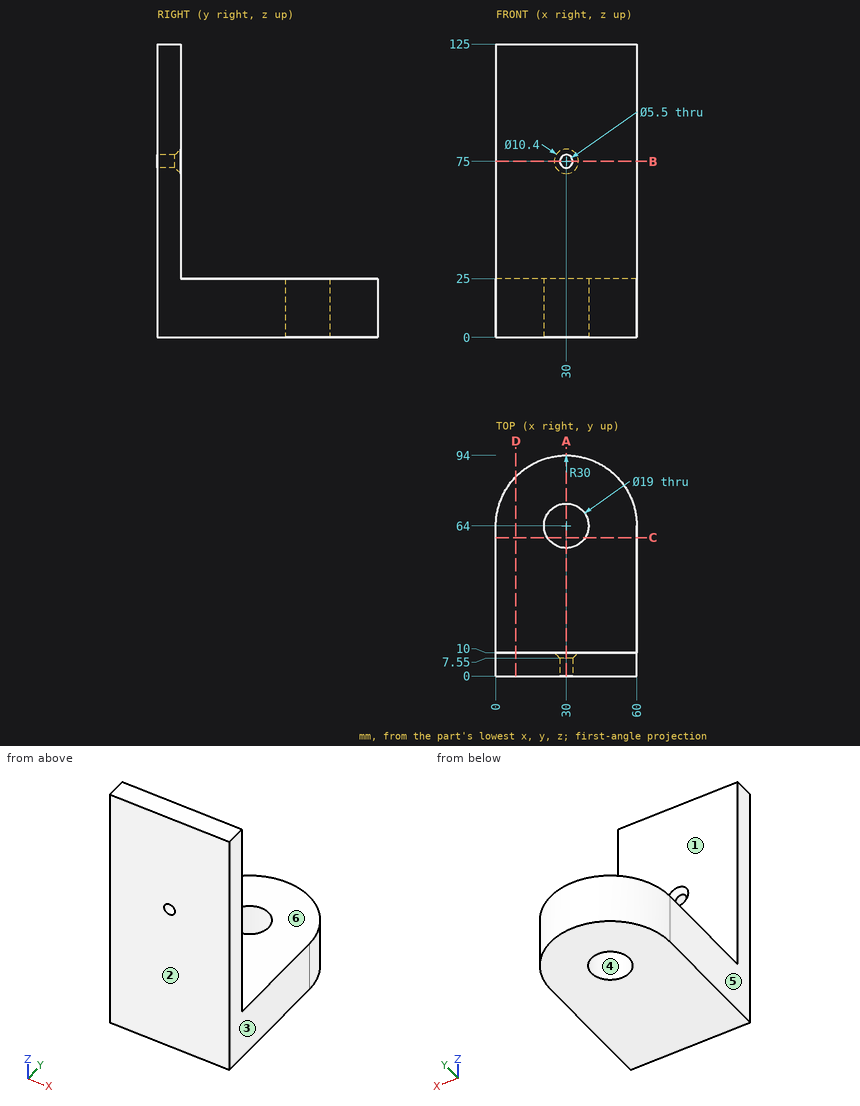
Input: dimensioned drawing with shaded views. Units: mm. Origin: part minimum x, y, z. A direction names the side the tool comes from. Round coordinates to 2 decimals unless told otherwise and drop trailing zeros. Order: outer loops, then holes, each group sorted by start corner. A loop starts at its lowest first (then second) coordinate and runs counter-clockwise, first axis right, second up.
1. Cut plane B-B, the plane z = 75. Output: boundary loops of the cut face in (x, y).
The answers:
outline: (0, 0) - (27.25, 0) - (27.25, 7.55) - (24.8, 10) - (0, 10) - close; (32.75, 0) - (60, 0) - (60, 10) - (35.2, 10) - (32.75, 7.55) - close
2. Cut plane C-C, the plane y = 59. Output: boundary loops of the cut face in (x, z), then the cut area to 3 significant figures.
The answers:
outline: (0, 0) - (21.92, 0) - (21.92, 25) - (0, 25) - close; (38.08, 0) - (60, 0) - (60, 25) - (38.08, 25) - close
area: 1,100 mm2
3. Pin query (flat end, axial travel): P1, Ø12, axis at x = 37.5, y = 82, coming from the +Z side; P2, Ø3, axis at x = 42.5, z = 53, coming from the +Y side; P3, Ø1.5, axis at x = 22, y = 51.5, coming from the -Z side; P4, Ø5, axis at y = 72.5, z = 18.5, coming from the +X side. Return the tip coordinate at first contact, or that it passes through.
The answers:
P1: stops at z = 25
P2: stops at y = 10
P3: stops at z = 0
P4: stops at x = 59.39
4. Mould query, pull axis Y, two halves, no side actions, for the marked faces 1, 2, 3 and 4. Classes: released by +Y, released by -Y, zero draft, split by the parting line, or undercut.
The answers:
face 1: released by +Y
face 2: released by -Y
face 3: zero draft
face 4: undercut
5. Cut plane D-D, the plane x = 8.5. Output: boundary loops of the cut face in (y, z), then the cut area to 3 significant figures.
The answers:
outline: (0, 0) - (84.92, 0) - (84.92, 25) - (10, 25) - (10, 125) - (0, 125) - close
area: 3,120 mm2
6. Set-up query: the marked faces 5 and 6. Return all of +Z, -Z, +X, -X, +Y, -Y with unobstructed straight access to the full face (end or side cutting, diameter ignored); none if empty.
The answers:
face 5: +Z, -Z, -X, +Y, -Y
face 6: +Z, +X, -X, +Y
7. Material intervals for line 1 (X direction, y = 2, z = 75); line 2 (Y direction, x = 30, z = 5); line 3 (Z direction, x = 30, y = 2.25), sorted ascending.
The answers:
line 1: x = 0 to 27.25, 32.75 to 60
line 2: y = 0 to 54.5, 73.5 to 94
line 3: z = 0 to 72.25, 77.75 to 125
8. Cut plane A-A, the plane x = 30. Output: boundary loops of the cut face in (y, z), then the cut area to 3 significant figures.
The answers:
outline: (0, 0) - (54.5, 0) - (54.5, 25) - (10, 25) - (10, 69.8) - (7.55, 72.25) - (0, 72.25) - close; (0, 77.75) - (7.55, 77.75) - (10, 80.2) - (10, 125) - (0, 125) - close; (73.5, 0) - (94, 0) - (94, 25) - (73.5, 25) - close
area: 2,810 mm2
